For this review, take the finished solid that the model builds, in its own axes (mm). A direction names the side the tool comes from. Give positions to 0.01 mm unless a question says otherwise; leave off trailing zeros. Order: outer loops, then holes, each group sorted by start corner. A loop starts at its lowest first (then second) coordinate and runs counter-clockwise, first axis right, second up. Notation, with made-up numbers: M 71,71 L 109,71 A33 ccw 109,108 Z; hole C 16,-5.75 d11. An arc over 180 degrees is marked long. Answer as CSV lines item,"result". Start each with the question number.
1. We need section B-B, the plane z = 172. Give the boundary of the cut face in (x, y) (3 decimals), and give its area (3 significant figures).
2. Machinability: for faces 1 (the flat face through (3.175, 42, 351)), 2 (the flat face through (2, 41, 711.2)), which of the approach directions +Z, -Z, +X, -X, +Y, -Y give a long, thin tool a straight path to every point of the face, cutting with its end or side? Answer none if there is none.
3. Clearance check with a flat-ended pin moving along its axis: P1, Ø5, axis at y = 48.5, z = 198.5, coming from the +X side (3 decimals). State where the tip first meets the part, or that it passes through.
4. We need section C-C, the plane y = 24. Give the boundary of the cut face in (x, z) (3 decimals), and give its area (3 significant figures).
5. We need section A-A, the plane x = 7. Give the boundary of the cut face in (y, z) (3 decimals), and give its area (3 significant figures).
6. For line 1 along Y through (x, z) = (8.75, 142) (3 decimals); line 2 along X through (y, z) = (25.5, 46.5) (3 decimals), list the stretches that pass through material, from the lowest coordinate up.
7. Mouldability with a two-part tool opening along Y and no side actions: class faces 3 (the flat face through (0, 42, 351)), 4 (the flat face through (13, 82.55, 351)), 5 (the flat face through (14, 3.175, 351)) as pulls with the +Y half, pulls with the -Y half, needs draft (parallel to the pull), parting line crosses it, or undercut.
Autodesk Inventor part; units mm, degrees
ref_plane "YZ Plane" through (0, 0, 0) normal (1, 0, 0) x (0, 1, 0)
ref_plane "XZ Plane" through (0, 0, 0) normal (0, 1, 0) x (-1, 0, 0)
ref_plane "XY Plane" through (0, 0, 0) normal (0, 0, 1) x (1, 0, 0)
sketch "Sketch1" plane through (0, 0, 0) normal (0, 0, 1) x (1, 0, 0)
  line L0 (0, 0) -> (25.4, 0)
  line L1 (25.4, 0) -> (25.4, 3.175)
  line L2 (3.175, 82.55) -> (0, 82.55)
  line L3 (0, 82.55) -> (0, 0)
  line L4 (3.175, 79.375) -> (3.175, 3.175)
  line L5 (3.175, 3.175) -> (25.4, 3.175)
  line L6 (3.175, 82.55) -> (25.4, 82.55)
  line L7 (25.4, 82.55) -> (25.4, 79.375)
  line L8 (25.4, 79.375) -> (3.175, 79.375)
  dimension "d0" = 82.55
  dimension "d1" = 25.4
  dimension "d2" = 3.175
  dimension "d3" = 3.175
  dimension "d6" = 3.175
  dimension "d7" = 25.4
extrude "Extrusion1" add sketch "Sketch1" along normal blind 711.2
equation "\"d3\" = d2"
equation "\"d6\" = d3"
equation "\"d7\" = d1"
properties part number "frame 7 outside U"
Result set:
1,outline,"M 0,0 L 25.4,0 L 25.4,3.175 L 3.175,3.175 L 3.175,79.375 L 25.4,79.375 L 25.4,82.55 L 0,82.55 Z"
1,area,"403 mm2"
2,face 1,"+Z, -Z, +X"
2,face 2,"+Z, +X, -X, +Y, -Y"
3,P1,"x = 3.175"
4,outline,"M 0,0 L 3.175,0 L 3.175,711.2 L 0,711.2 Z"
4,area,"2,260 mm2"
5,outline,"M 0,0 L 3.175,0 L 3.175,711.2 L 0,711.2 Z; M 79.375,0 L 82.55,0 L 82.55,711.2 L 79.375,711.2 Z"
5,area,"4,520 mm2"
6,line 1,"0 to 3.175, 79.375 to 82.55"
6,line 2,"0 to 3.175"
7,face 3,"needs draft"
7,face 4,"pulls with the +Y half"
7,face 5,"undercut"
